from build123d import *

# Parameters (mm, degrees)
F1_DEPTH = 12.7
F2_R     = 6.35
F3_DEPTH = 25.4
F4_R     = 6.35
F5_DEPTH = 25.4
F6_R     = 25.4
F7_DEPTH = 25.4
F8_W     = 50.8
F8_H     = 12.7
F8_H_2   = 12.700023
F8_W_2   = 12.7
F8_H_3   = 50.8
F9_DEPTH = 25.4


with BuildPart() as f1:
    # F0 (on Top) → F1 (new body)
    with BuildSketch(Plane.XY):
        with BuildLine():
            Line((-333.067566, -685.8), (333.067566, -685.8))
            ThreePointArc((333.067566, -685.8), (356.467306, -675.046359), (368.3, -652.173317))
            Line((368.3, -652.173317), (368.3, 662.494829))
            ThreePointArc((368.3, 662.494829), (360.848675, 678.418518), (345.550371, 687.081542))
            ThreePointArc((345.550371, 687.081542), (224.27561, 745.924123), (166.778415, 867.842495))
            Line((166.778415, 867.842495), (166.778415, 1012.140632))
            ThreePointArc((166.778415, 1012.140632), (138.228781, 1103.662105), (50.8, 1143))
            Line((50.8, 1143), (0, 1143))
            Line((0, 1143), (-50.8, 1143))
            ThreePointArc((-50.8, 1143), (-138.228781, 1103.662105), (-166.778415, 1012.140632))
            Line((-166.778415, 1012.140632), (-166.778415, 867.842495))
            ThreePointArc((-166.778415, 867.842495), (-224.27561, 745.924123), (-345.550371, 687.081542))
            ThreePointArc((-345.550371, 687.081542), (-360.848675, 678.418518), (-368.3, 662.494829))
            Line((-368.3, 662.494829), (-368.3, -652.173317))
            ThreePointArc((-368.3, -652.173317), (-356.467306, -675.046359), (-333.067566, -685.8))
        make_face()
    extrude(amount=F1_DEPTH)

    # F2 (on face) → F3 (cut)
    with BuildSketch(Plane.XY.offset(12.7)):
        with Locations((0, 1012.140632)):
            Circle(F2_R)
    extrude(amount=-F3_DEPTH, mode=Mode.SUBTRACT)

    # F4 (on face) → F5 (cut)
    with BuildSketch(Plane.XY.offset(12.7)):
        with Locations((-203.2, -609.6)):
            Circle(F4_R)
        with Locations((203.2, -609.6)):
            Circle(F4_R)
    extrude(amount=-F5_DEPTH, mode=Mode.SUBTRACT)

    # F6 (on face) → F7 (cut)
    with BuildSketch(Plane.XY.offset(12.7)):
        with Locations((0, 687.081542)):
            Circle(F6_R)
    extrude(amount=-F7_DEPTH, mode=Mode.SUBTRACT)

    # F8 (on face) → F9 (cut)
    with BuildSketch(Plane.XY.offset(12.7)):
        with Locations((0, -558.8)):
            Rectangle(F8_W, F8_H)
        with Locations((-203.2, -558.800011)):
            Rectangle(F8_W, F8_H_2)
        with Locations((203.2, -558.800011)):
            Rectangle(F8_W, F8_H_2)
        with Locations((-222.25, -323.85)):
            Rectangle(F8_W_2, F8_H_3)
        with Locations((222.25, -323.85)):
            Rectangle(F8_W_2, F8_H_3)
    extrude(amount=-F9_DEPTH, mode=Mode.SUBTRACT)


solid = f1.part
The model under review builds one solid part; all positions refer to its coordinate system, in mm. Round coordinates to 2 decimals unless told otherwise and drop trailing zeros. Loops run counter-clockwise (first coordinate to the right, second up) from the corner with the lowest first, then second, coordinate; pieces in that order, holes last. Notation, with made-up numbers: (19.25, -38) -> (26.25, -38) arc R8 ccw to (26.25, -23) -> close; hole circle Ø1 at (12.5, 21). An arc over 180 degrees is marked (long way). Answer as CSV lines item,"result".
1) For P1, Ø5, axis at x = 192, z = 2, coming from the +Y side; P2, Ø6.5, axis at x = 221, z = 4.5, coming from the +Y side; P3, Ø4, axis at x = 199, z = 5, coming from the +Y side; P4, Ø8, axis at x = -101, y = -123, coming from the -Z side, all flat-tipped, find the tip position at first contact; note any pin that passes through.
Geometry results:
P1,"stops at y = 793.17"
P2,"stops at y = 752.84"
P3,"stops at y = 780.25"
P4,"stops at z = 0"
2) To check wall thickness, follow line 1 along Y through (x, z) = (0, 3); line 2 along X through (y, z) = (-609.6, 4); line 3 along X through (y, z) = (-553, 10.75). State the ranges of each line that lie inside material, in increasing order. Write a range as from..to.
Geometry results:
line 1,"y = -685.8..-565.15, -552.45..661.68, 712.48..1005.79, 1018.49..1143"
line 2,"x = -368.3..-209.55, -196.85..196.85, 209.55..368.3"
line 3,"x = -368.3..-228.6, -177.8..-25.4, 25.4..177.8, 228.6..368.3"
3) Add section B-B on y = 925. Write out the cut boundary in (x, z).
Geometry results:
outline,"(-166.78, 0) -> (166.78, 0) -> (166.78, 12.7) -> (-166.78, 12.7) -> close"
4) Add section A-A on z = 2.75. State how many separate pieces and enclosed holes the cut face has, plus the area to 3 significant figures.
Geometry results:
separate pieces,"1"
enclosed holes,"9"
area,"1,170,000 mm²"
5) Draft analysis for pull direction Y (two halves, no side actions). For faces 1 (the face through (-5, 241, 12.7)), 2 (the face through (-3.307, 712.265, 6.439)), 3 (the face through (356.2, -675.3, 6.3)), state which applies: pulls with the +Y half, pulls with the -Y half, needs draft (parallel to the pull), parting line crosses it, or undercut.
Geometry results:
face 1,"needs draft"
face 2,"undercut"
face 3,"pulls with the -Y half"
